Read the model definition and answer for the solid it produces. Units are mm, in the model's axes. Face numbers are marked on the shaded views. A direction names the side the tool comes from. Coordinates: 2 decimals unless noted, no trailing zeros. Order: outer loops, then holes, each group sorted by start corner. A loop starts at its lowest first (then second) coordinate and runs counter-clockwise, first axis right, second up. Notation, with made-up numbers: (56, -26.75) - (74, -26.75) arc R24 cw to (74, 3.25) - close; hole circle Ø8 at (68, 46). An arc over 180 degrees is marked (long way). Answer as a JSON object with one key per item and string values. Group by question number.
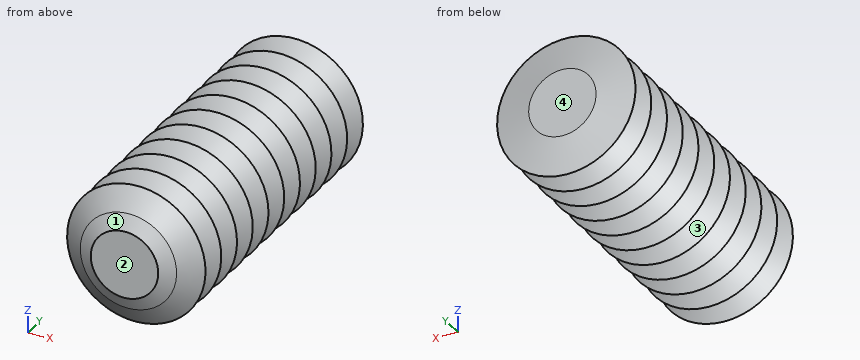
from build123d import *


with BuildPart() as part:
    # Sketch1 → Elemento_elastico_en_serie (revolve)
    with BuildSketch(Plane.XY, mode=Mode.PRIVATE) as elemento_elastico_en_serie_sk:
        Polygon((0, 0), (2.24, 0), (4.6, -0.5), (3.2, -1.5), (4.6, -2.5), (3.2, -3.5), (4.6, -4.5), (3.2, -5.5), (4.6, -6.5), (3.2, -7.5), (4.6, -8.5), (3.2, -9.5), (4.6, -10.5), (3.2, -11.5), (4.6, -12.5), (3.2, -13.5), (4.6, -14.5), (3.2, -15.5), (4.6, -16.5), (3.2, -17.5), (4.6, -18.5), (3.2, -19.5), (4.6, -20.5), (3.2, -21.5), (2.24, -22), (0, -22), align=None)
    revolve(elemento_elastico_en_serie_sk.sketch.rotate(Axis((0, -26, 0), (0, 1, 0)), 90), axis=Axis((0, -26, 0), (0, 1, 0)))


solid = part.part
1. For a pull along X with two mould halves and no side action, classify the marked faces 1 and 2 as pulls with the +X half, pulls with the -X half, needs draft (parallel to the pull), parting line crosses it, or undercut.
2. Given pin 1 (1.5 mm diameter, centred on x = -1.5, y = -3.5, fed in from -Z); pin 2 (4 mm diameter, centred on x = 0, y = -15, fed in from +Z); pin 3 (1 mm diameter, centred on y = -19, z = -2.5, fed in from +X), each flat-ended and moving along its own axis, determine where each tip first touches the part or whether it passes through.
3. Straight lines are drawn through the part: L1, parallel to Z at x = -2.75, y = -16.25; L2, parallel to Y at x = -1.75, z = -1.5; L3, parallel to X at y = -20.25, z = -2.5. For each, find the intervals that lie inside material, in ascending order.
4. For the marked faces 3 and 4, determine the directions among +Z, -Z, +X, -X, +Y, -Y from which every point of the face is accessible in a straight line to the end or side of a thin tool.
5. A cutting plane is placed at B-B on y = -19.25. Write down the section's boundary in (x, z), and give its area (3 significant figures).
Derived:
{
 "1": {"face 1": "parting line crosses it", "face 2": "needs draft"},
 "2": {"pin 1": "stops at z = -4.01", "pin 2": "stops at z = 4.6", "pin 3": "stops at x = 3.92"},
 "3": {"L1": "z = -3.24 to 3.24", "L2": "y = -21.97 to -0.01", "L3": "x = -3.44 to 3.44"},
 "4": {"face 3": "none", "face 4": "+Z, -Z, +X, -X, +Y"},
 "5": {"outline": "circle Ø7.1 at (0, 0)", "area": "39.6 mm2"}
}
